Verification items for the finished model (mm, model axes). A direction names the side the tool comes from. Coordinates: 2 decimals unless noted, no trailing zeros. Loops run counter-clockwise (first coordinate to the right, second up) from the corner with the lowest first, then second, coordinate; pieces in that order, holes last. Notation, with made-up numbers: (-19, 25.25) - (4, 25.25) arc R8 cw to (4, 40.25) - close; hole circle Ø6 at (-7.5, -32.75). An arc over 180 degrees is marked (long way). One line per item, written item: value. Start each with the question number.
(1) Section check B-B (z = 3). Record the boundary of the cut face in (x, y) (3 decimals).
(2) Gauge pin test, flat ends, axial feed: P1, Ø3, axis at x = 45, z = 4, coming from the +Y side; P2, Ø0.5, axis at x = -1, y = 10.5, coming from the +Z side; P3, Ø3, axis at y = -10.5, z = 3.5, coming from the +X side. Record the tip position at first contact, or that the pin passes through.
(3) Section check D-D (x = 34). Record the boundary of the cut face in (y, z), plus the area to 3 significant figures.
(4) Section check A-A (x = 0). Record the boundary of the cut face in (y, z).
(5) Set-up check for faces 5 (the face through (0, 6, 6.34)), 6 (the face through (3.1, 6.8, 8.3)), 7 (the face through (0, -17.68, 3)): record each of +Z, -Z, +X, -X, +Y, -Y from which the full face is reachable in a straight line by a thin tool's end or side.
(6) Thickness scan on probe 1 along Y at (x, z) = (0, 7.5); probe 2 along Y at (x, z) = (39, 4); probe 3 along Z at (x, y) = (18.5, -18). Record the ranges inside material, lowest first. Write a range as [from, to].
(7) Section check C-C (y = 2). Record the boundary of the cut face in (x, z).
(8) Draft check along Y on faces 1 (the face through (0, 6.82, 3)), 2 (the face through (40, -17.68, 3)), 3 (the face through (11, -3, 0)), 4 (the face through (-11.725, -7.228, 3.126)). Enter one of: +Y half, -Y half, draft (parallel to the pull), parting line (faces both ways), or undercut.
```python
from build123d import *
from build123d.topology import SkipClean

# Parameters (mm, degrees)
BOSS_EXTRUDE1_DEPTH = 6.34
SKETCH6_R           = 7.235705293
SKETCH6_R_2         = 3.175
BOSS_EXTRUDE2_DEPTH = 1.96
SKETCH8_W           = 6.34
SKETCH8_H           = 4
BOSS_EXTRUDE4_DEPTH = 35


with BuildPart() as part:
    # Sketch1 → Boss-Extrude1 (new body)
    # profile 1 of 5: a face of its own
    with BuildSketch(Plane.XY):
        with BuildLine():
            ThreePointArc((7.235705293, 8.31996617), (0, 15.555671463), (-7.235705293, 8.31996617))
            ThreePointArc((-7.235705293, 8.31996617), (-6.76521969, 5.753405509), (-5.414947438, 3.520614617))
            Line((-5.414947438, 3.520614617), (-3.113806984, 7.440196422))
            ThreePointArc((-3.113806984, 7.440196422), (0, 11.555671463), (3.113806984, 7.440196422))
            Line((3.113806984, 7.440196422), (5.414947438, 3.520614617))
            ThreePointArc((5.414947438, 3.520614617), (6.76521969, 5.753405509), (7.235705293, 8.31996617))
        make_face()
    # profile 2 of 5: a face of its own
    with BuildSketch(Plane.XY):
        with BuildLine():
            Line((-7.235705293, 8.31996617), (-22.5, -17.68003383))
            Line((-22.5, -17.68003383), (-22.5, -21.68003383))
            Line((-22.5, -21.68003383), (22.5, -21.68003383))
            Line((22.5, -21.68003383), (22.5, -17.68003383))
            Line((22.5, -17.68003383), (7.235705293, 8.31996617))
            ThreePointArc((7.235705293, 8.31996617), (6.76521969, 5.753405509), (5.414947438, 3.520614617))
            Line((5.414947438, 3.520614617), (17.861599202, -17.68003383))
            Line((17.861599202, -17.68003383), (-17.861599202, -17.68003383))
            Line((-17.861599202, -17.68003383), (-5.414947438, 3.520614617))
            ThreePointArc((-5.414947438, 3.520614617), (-6.76521969, 5.753405509), (-7.235705293, 8.31996617))
        make_face()
    # profile 3 of 5: a face of its own
    with BuildSketch(Plane.XY):
        with BuildLine():
            Line((-3.113806984, 7.440196422), (-5.414947438, 3.520614617))
            ThreePointArc((-5.414947438, 3.520614617), (0, 1.084260877), (5.414947438, 3.520614617))
            Line((5.414947438, 3.520614617), (3.113806984, 7.440196422))
            ThreePointArc((3.113806984, 7.440196422), (0, 11.555671463), (-3.113806984, 7.440196422))
        make_face()
        with BuildLine():
            ThreePointArc((-2.798325392, 6.81996617), (-3.175, 8.31996617), (-2.798325392, 9.81996617))
            ThreePointArc((-2.798325392, 9.81996617), (0, 11.49496617), (2.798325392, 9.81996617))
            ThreePointArc((2.798325392, 9.81996617), (3.079391833, 9.093251978), (3.175, 8.31996617))
            ThreePointArc((3.175, 8.31996617), (3.079391833, 7.546680362), (2.798325392, 6.81996617))
            ThreePointArc((2.798325392, 6.81996617), (0, 5.14496617), (-2.798325392, 6.81996617))
        make_face(mode=Mode.SUBTRACT)
    # profile 4 of 5: a face of its own
    with BuildSketch(Plane.XY):
        with BuildLine():
            Line((2.798325392, 6.81996617), (-2.798325392, 6.81996617))
            ThreePointArc((-2.798325392, 6.81996617), (0, 5.14496617), (2.798325392, 6.81996617))
        make_face()
    # profile 5 of 5: a face of its own
    with BuildSketch(Plane.XY):
        with BuildLine():
            ThreePointArc((2.798325392, 9.81996617), (0, 11.49496617), (-2.798325392, 9.81996617))
            Line((-2.798325392, 9.81996617), (2.798325392, 9.81996617))
        make_face()
    extrude(amount=BOSS_EXTRUDE1_DEPTH)

    # Sketch6 → Boss-Extrude2 (add)
    with SkipClean():  # the faces are left unmerged after this step: merging them gives an invalid solid
        with BuildSketch(Plane.XY.offset(6.34)):
            with Locations((0, 8.31996617)):
                Circle(SKETCH6_R)
            with Locations(Location((0, 8.31996617, 0), (0, 0, 151.807139439))):
                Circle(SKETCH6_R_2, mode=Mode.SUBTRACT)
        extrude(amount=BOSS_EXTRUDE2_DEPTH)

    # Sketch8 → Boss-Extrude4 (add)
    with SkipClean():  # the faces are left unmerged after this step: merging them gives an invalid solid
        with BuildSketch(Plane(origin=(22.5, 0, 0), x_dir=(0, 0, -1), z_dir=(1, 0, 0))):
            with Locations((-3.17, -19.68003383)):
                Rectangle(SKETCH8_W, SKETCH8_H)
        extrude(amount=BOSS_EXTRUDE4_DEPTH)


solid = part.part
```
Responses:
1. outline: (-22.5, -21.68) - (57.5, -21.68) - (57.5, -17.68) - (22.5, -17.68) - (7.236, 8.32) arc R7.236 ccw to (-7.236, 8.32) - (-22.5, -17.68) - close; hole (-17.862, -17.68) - (17.862, -17.68) - (5.415, 3.521) arc R7.236 cw to (-5.415, 3.521) - close; hole (-2.798, 6.82) - (2.798, 6.82) arc R3.175 ccw to (2.798, 9.82) - (-2.798, 9.82) arc R3.175 ccw to start
2. P1: stops at y = -17.68
2. P2: stops at z = 6.34
2. P3: stops at x = 19.17
3. outline: (-21.68, 0) - (-17.68, 0) - (-17.68, 6.34) - (-21.68, 6.34) - close
3. area: 25.4 mm²
4. outline: (-21.68, 0) - (-17.68, 0) - (-17.68, 6.34) - (-21.68, 6.34) - close; (1.08, 0) - (6.82, 0) - (6.82, 6.34) - (5.14, 6.34) - (5.14, 8.3) - (1.08, 8.3) - close; (9.82, 0) - (15.56, 0) - (15.56, 8.3) - (11.49, 8.3) - (11.49, 6.34) - (9.82, 6.34) - close
5. face 5: +Z
5. face 6: +Z, +X, -X, +Y, -Y
5. face 7: +Z, -Z
6. probe 1: y = [1.08, 5.14], [11.49, 15.56]
6. probe 2: y = [-21.68, -17.68]
6. probe 3: z = [0, 6.34]
7. outline: (-10.95, 0) - (-6.31, 0) - (-6.31, 6.34) - (-10.95, 6.34) - close; (-3.52, 0) - (3.52, 0) - (3.52, 8.3) - (-3.52, 8.3) - close; (6.31, 0) - (10.95, 0) - (10.95, 6.34) - (6.31, 6.34) - close
8. face 1: undercut
8. face 2: +Y half
8. face 3: draft
8. face 4: undercut
